CAD build for the part. Positions are in the model's coordinates, mm. A direction names the side the tool comes from. Round coordinates to 2 decimals unless told otherwise and drop trailing zeros. Order: outer loops, then holes, each group sorted by start corner. A loop starts at its lowest first (then second) coordinate and runs counter-clockwise, first axis right, second up. Notation, with made-up numbers: M 29.25,74.5 L 55.25,74.5 A19 cw 55.25,108.5 Z; hole C 44,82 d1. An arc over 180 degrees is marked long. Put each result on its own line as item: value.
```python
from build123d import *

# Parameters (mm, degrees)
ESBO_O2_W                = 20
ESBO_O2_H                = 20
RESSALTO_EXTRUS_O1_DEPTH = 65
ESBO_O3_R                = 3.3
CORTE_EXTRUS_O1_DEPTH    = 67.520673478
ESBO_O4_R                = 3.3
CORTE_EXTRUS_O2_DEPTH    = 69.738635424
FILETE1_R                = 5
FILETE2_R                = 5
FILETE3_R                = 5
FILETE4_R                = 5
ESBO_O7_W                = 10
ESBO_O7_H                = 5
CORTE_EXTRUS_O3_DEPTH    = 69.738635424


with BuildPart() as part:
    # Esboço2 → Ressalto-extrusão1 (new body)
    with BuildSketch(Plane.XY):
        Rectangle(ESBO_O2_W, ESBO_O2_H)
    extrude(amount=RESSALTO_EXTRUS_O1_DEPTH)

    # Esboço3 → Corte-extrusão1 (cut, through all)
    with BuildSketch(Plane.XY.offset(65)):
        Circle(ESBO_O3_R)
    extrude(amount=-CORTE_EXTRUS_O1_DEPTH, mode=Mode.SUBTRACT)

    # Esboço4 → Corte-extrusão2 (cut, through all)
    with BuildSketch(Plane(origin=(0, -10, 0), x_dir=(-1, 0, 0), z_dir=(0, -1, 0))):
        with Locations(Location((0, -5, 0), (0, 0, 90))):
            Circle(ESBO_O4_R)
    extrude(amount=-CORTE_EXTRUS_O2_DEPTH, mode=Mode.SUBTRACT)

    # Filete1
    filete1_edges = [part.edges().sort_by_distance(p)[0] for p in [
        (10, -10, 32.5),
    ]]
    fillet(filete1_edges, radius=FILETE1_R)

    # Filete2
    filete2_edges = [part.edges().sort_by_distance(p)[0] for p in [
        (10, 10, 32.5),
    ]]
    fillet(filete2_edges, radius=FILETE2_R)

    # Filete3
    filete3_edges = [part.edges().sort_by_distance(p)[0] for p in [
        (-10, 10, 32.5),
    ]]
    fillet(filete3_edges, radius=FILETE3_R)

    # Filete4
    filete4_edges = [part.edges().sort_by_distance(p)[0] for p in [
        (-10, -10, 32.5),
    ]]
    fillet(filete4_edges, radius=FILETE4_R)

    # Esboço7 → Corte-extrusão3 (cut, through all)
    with BuildSketch(Plane(origin=(0, -10, 0), x_dir=(-1, 0, 0), z_dir=(0, -1, 0))):
        with Locations((0, -52.5)):
            Rectangle(ESBO_O7_W, ESBO_O7_H)
    extrude(amount=-CORTE_EXTRUS_O3_DEPTH, mode=Mode.SUBTRACT)


solid = part.part
```
Item 1: Mould opens along Z. For faces 1 (the flat face through (5, 0, 53)), 2 (the cylindrical face through (-0.43, 3.27, 27.82)), 3 (the flat face through (0, 5, 0)) say: pulls with the +Z half, pulls with the -Z half, needs draft (parallel to the pull), parting line crosses it, or undercut.
Answers below:
face 1: undercut
face 2: needs draft
face 3: pulls with the -Z half
Item 2: Probe line 1 along Z through (x, y) = (0, -5.75); line 2 along Z through (x, y) = (-3.5, 3.5); line 3 along Y through (x, z) = (0, 40.5). List the from-to ranges inside material, lowest first. Write a range as [from, to].
Answers below:
line 1: [0, 1.7], [8.3, 50], [55, 65]
line 2: [0, 50], [55, 65]
line 3: [-10, -3.3], [3.3, 10]
Item 3: Band-saw the part on D-D on x = -2. Give the cut face in (y, z), and give its area (3 significant figures).
Answers below:
outline: M -10,0 L -2.62,0 L -2.62,2.38 L -10,2.38 Z; M -10,7.62 L -2.62,7.62 L -2.62,50 L -10,50 Z; M -10,55 L -2.62,55 L -2.62,65 L -10,65 Z; M 2.62,0 L 10,0 L 10,2.38 L 2.62,2.38 Z; M 2.62,7.62 L 10,7.62 L 10,50 L 2.62,50 Z; M 2.62,55 L 10,55 L 10,65 L 2.62,65 Z
area: 808 mm²
Item 4: Band-saw the part on A-A on z = 14. Give the cut face in (x, y).
Answers below:
outline: M -10,-5 A5 ccw -5,-10 L 5,-10 A5 ccw 10,-5 L 10,5 A5 ccw 5,10 L -5,10 A5 ccw -10,5 Z; hole C 0,0 d6.6
Item 5: Tool access for faces 4 (the cylindrical face through (9, 8, 33)), 5 (the flat face through (3, 2, 55)): list every direction of +Z, -Z, +X, -X, +Y, -Y with a clear straight run to the whole face (end or side of a thin tool).
Answers below:
face 4: +Z, -Z, +X, +Y
face 5: +Y, -Y
Item 6: Band-saw the part on B-B on x = 4.25. Give the cut face in (y, z), and give its area (3 significant figures).
Answers below:
outline: M -10,0 L 10,0 L 10,50 L -10,50 Z; M -10,55 L 10,55 L 10,65 L -10,65 Z
area: 1,200 mm²
Item 7: Band-saw the part on C-C on y = -6. Give the cut face in (x, z).
Answers below:
outline: M -9.9,0 L 9.9,0 L 9.9,65 L -9.9,65 Z; hole M -5,50 L 5,50 L 5,55 L -5,55 Z; hole C 0,5 d6.6
Item 8: Pin check, flat tip, straight feed: P1, Ø3, axis at x = -7.5, z = 13.5, coming from the -Y side. Stop position of the tip, or through.
Answers below:
P1: y = -9.9
